Job drawing, mm, ordinate dimensions from the low corner. One solid piece. A direction names the side the tool comes from. Round coordinates to 2 decimals unless told otherwise and drop trailing zeros. Write each loop counter-clockwise with the first axis right and the second up, starting at its lowest first coordinate (ties: lowest second). Pieces come first, ordered by that corner, then holes. Notation, with made-up numbers: (25.5, 46.25) -> (74.5, 46.25) arc R5 ccw to (74.5, 50.25) -> close; hole circle Ø9 at (47, 28). An arc over 180 degrees is marked (long way). Use CSV: the item, a comma, the result in double quotes. Start each with the question number.
(1) Saw through at B-B (z = 21). Give the cut face in (x, y).
(2) Saw through at C-C (x = 34). Give the cut face in (y, z) (3 decimals).
(3) Two-plate mould, pull along X, no slides. Class the marked faces 5, 6 and 7: released by +X, released by -X, zero draft, split by the parting line, or undercut.
(4) Which spindle directions (+Z, -Z, +X, -X, +Y, -Y) get a long thin tool onto all of the face, cutting with end or side? Do the marked faces 1, 2, 3 and 4. Say none if no direction does.
(5) Probe line 1 (X direction, y = 4.5, z = 4); line 2 (X direction, y = 17.75, z = 19.5); line 3 (X direction, y = 13.75, z = 25.5). List the from-to ranges inside material, lowest first. Write a range as [from, to].
(6) Saw through at A-A (y = 7.75). Give the cut face in (x, z) (3 decimals), plus the area to 3 significant figures.
(7) Drop flat-ended pins along their axis: pin 1 (1.5 mm diameter, centred on x = 2, y = 16.5, fed in from -Z); pin 2 (3 mm diameter, centred on x = 14, y = 15.5, fed in from -Z); pin 3 (5.5 mm diameter, centred on y = 15.5, z = 25, fed in from +X). Give the stop position or say it passes through.
(8) Saw through at D-D (z = 8). Give the cut face in (x, y), plus the area to 3 significant figures.
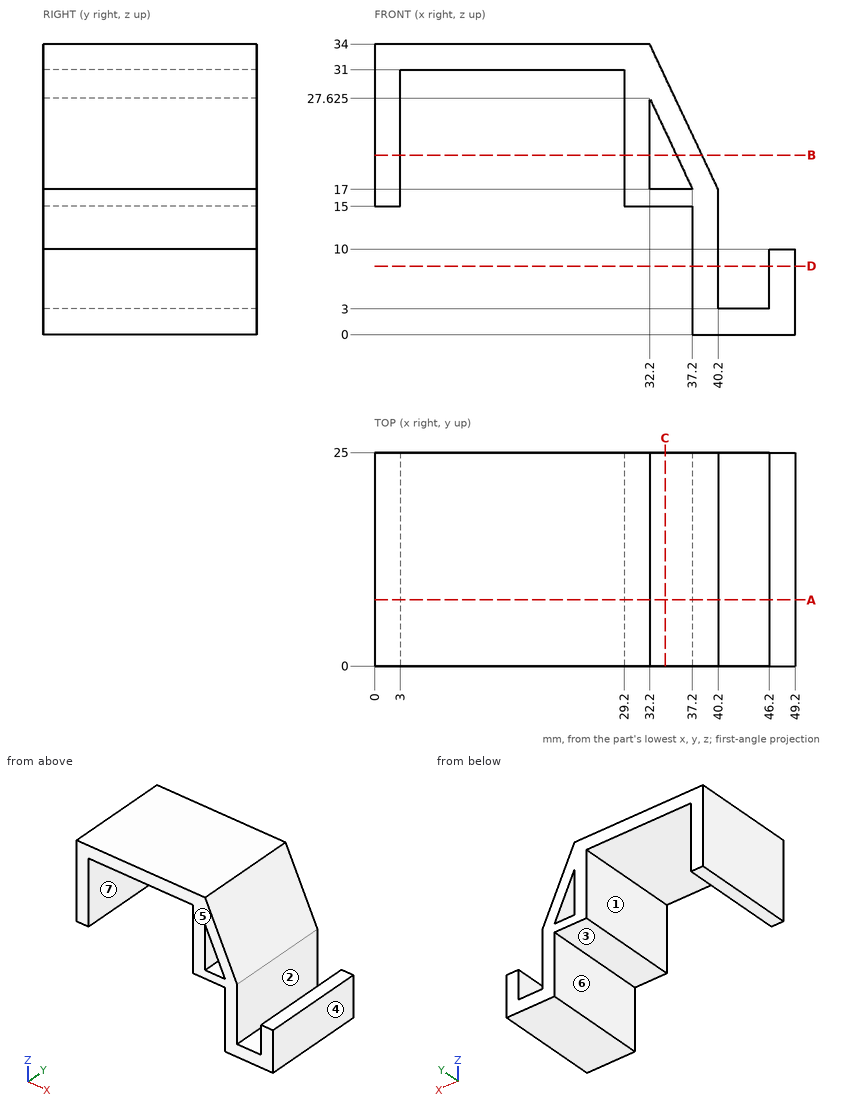
Answers:
1,outline,"(0, 0) -> (3, 0) -> (3, 25) -> (0, 25) -> close; (29.2, 0) -> (32.2, 0) -> (32.2, 25) -> (29.2, 25) -> close; (35.32, 0) -> (38.32, 0) -> (38.32, 25) -> (35.32, 25) -> close"
2,outline,"(0, 15) -> (25, 15) -> (25, 17) -> (0, 17) -> close; (0, 23.8) -> (25, 23.8) -> (25, 30.175) -> (0, 30.175) -> close"
3,face 5,"zero draft"
3,face 6,"released by -X"
3,face 7,"undercut"
4,face 1,"-Z, +Y, -Y"
4,face 2,"+Z, +Y, -Y"
4,face 3,"-Z, -X, +Y, -Y"
4,face 4,"+Z, -Z, +X, +Y, -Y"
5,line 1,"x = [37.2, 40.2], [46.2, 49.2]"
5,line 2,"x = [0, 3], [29.2, 32.2], [36.02, 39.02]"
5,line 3,"x = [0, 3], [29.2, 32.2], [33.2, 36.2]"
6,outline,"(0, 15) -> (3, 15) -> (3, 31) -> (29.2, 31) -> (29.2, 15) -> (37.2, 15) -> (37.2, 0) -> (49.2, 0) -> (49.2, 10) -> (46.2, 10) -> (46.2, 3) -> (40.2, 3) -> (40.2, 17) -> (32.2, 34) -> (0, 34) -> close; hole (32.2, 17) -> (37.2, 17) -> (32.2, 27.625) -> close"
6,area,"343 mm²"
7,pin 1,"stops at z = 15"
7,pin 2,"stops at z = 31"
7,pin 3,"stops at x = 37.73"
8,outline,"(37.2, 0) -> (40.2, 0) -> (40.2, 25) -> (37.2, 25) -> close; (46.2, 0) -> (49.2, 0) -> (49.2, 25) -> (46.2, 25) -> close"
8,area,"150 mm²"
